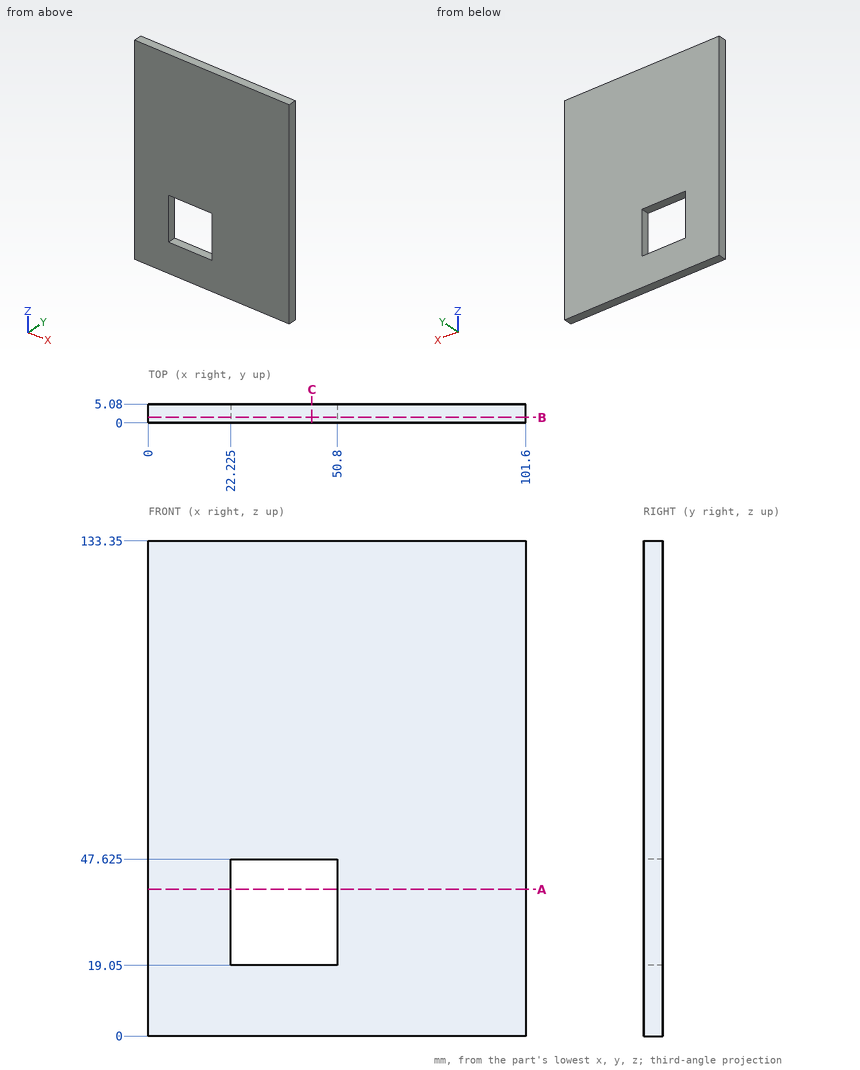
Part print with two shaded views. Sizes in mm from the minimum x, y, z corner. Coordinates: 2 decimals unless noted, no trailing zeros. Order: outer loops, then holes, each group sorted by start corner. A loop starts at its lowest first (then second) coordinate and runs counter-clockwise, first axis right, second up. Notation, with made-up numbers: M 3.5,20 L 61.5,20 A26 cw 61.5,38 Z; hole C -35,69 d6. An arc over 180 degrees is marked long. Use a Markdown table: item, result.
(1) Cut at B-B on y = 1.5. Write the cut outline in (x, z) (3 decimals), then the cut area to 3 significant figures.
A:
| item | result |
|---|---|
| outline | M 0,0 L 101.6,0 L 101.6,133.35 L 0,133.35 Z; hole M 22.225,19.05 L 50.8,19.05 L 50.8,47.625 L 22.225,47.625 Z |
| area | 12,700 mm^2 |
(2) Cut at A-A on z = 39.5. Write the cut outline in (x, y) (3 decimals).
A:
| item | result |
|---|---|
| outline | M 0,0 L 22.225,0 L 22.225,5.08 L 0,5.08 Z; M 50.8,0 L 101.6,0 L 101.6,5.08 L 50.8,5.08 Z |
(3) Probe L1, parallel to X at y = 4.6, z = 22.5 (3 decimals); L2, parallel to Z at x = 50, y = 2.1 (3 decimals). List the from-to ranges inside material, lowest first.
A:
| item | result |
|---|---|
| L1 | x = 0 to 22.225, 50.8 to 101.6 |
| L2 | z = 0 to 19.05, 47.625 to 133.35 |
(4) Cut at C-C on x = 44. Write the cut outline in (y, z) (3 decimals).
A:
| item | result |
|---|---|
| outline | M 0,0 L 5.08,0 L 5.08,19.05 L 0,19.05 Z; M 0,47.625 L 5.08,47.625 L 5.08,133.35 L 0,133.35 Z |
